```python
from build123d import *

# Parameters (mm, degrees)
BOSS_EXTRUDE1_DEPTH = 10.5
SKETCH4_W           = 30.5
SKETCH4_H           = 6
BOSS_EXTRUDE2_DEPTH = 5
SKETCH5_W           = 30.5
SKETCH5_H           = 6
BOSS_EXTRUDE3_DEPTH = 6
SKETCH6_R           = 6
CUT_EXTRUDE2_DEPTH  = 5
SKETCH11_W          = 30.5
SKETCH11_H          = 6
BOSS_EXTRUDE5_DEPTH = 15
CUT_EXTRUDE4_DEPTH  = 31.5


with BuildPart() as part:
    # Sketch2 → Boss-Extrude1 (new body)
    with BuildSketch(Plane(origin=(0, 0, 0), x_dir=(0, 0, -1), z_dir=(1, 0, 0))):
        with BuildLine():
            Line((2.711841856, 20.960264901), (-3.288158144, 20.960264901))
            Line((-3.288158144, 20.960264901), (-3.288158144, 11.676412171))
            ThreePointArc((-3.288158144, 11.676412171), (-14.220841983, 11.857208885), (-15.122437882, 0.960264901))
            Line((-15.122437882, 0.960264901), (-33.288158144, 0.960264901))
            Line((-33.288158144, 0.960264901), (-33.288158144, -5.039735099))
            Line((-33.288158144, -5.039735099), (2.711841856, -5.039735099))
            Line((2.711841856, -5.039735099), (2.711841856, 20.960264901))
        make_face()
    extrude(amount=-BOSS_EXTRUDE1_DEPTH)

    # Sketch4 → Boss-Extrude2 (add)
    with BuildSketch(Plane(origin=(0, 20.960264901, 0), x_dir=(1, 0, 0), z_dir=(0, 1, 0))):
        with Locations((4.75, -0.288158144)):
            Rectangle(SKETCH4_W, SKETCH4_H)
    extrude(amount=BOSS_EXTRUDE2_DEPTH)

    # Sketch5 → Boss-Extrude3 (add)
    with BuildSketch(Plane.XY.offset(33.288158144)):
        with Locations((4.75, -2.039735099)):
            Rectangle(SKETCH5_W, SKETCH5_H)
    extrude(amount=BOSS_EXTRUDE3_DEPTH)

    # Sketch6 → Cut-Extrude2 (cut)
    with BuildSketch(Plane(origin=(0, 0, 0), x_dir=(0, 0, -1), z_dir=(1, 0, 0))):
        with Locations((-8.806939463, 5.923867659)):
            Circle(SKETCH6_R)
    extrude(amount=-CUT_EXTRUDE2_DEPTH, mode=Mode.SUBTRACT)

    # Sketch11 → Boss-Extrude5 (add)
    with BuildSketch(Plane(origin=(0, 0.960264901, 0), x_dir=(1, 0, 0), z_dir=(0, 1, 0))):
        with Locations((4.75, -36.288158144)):
            Rectangle(SKETCH11_W, SKETCH11_H)
    extrude(amount=BOSS_EXTRUDE5_DEPTH)

    # Sketch12 → Cut-Extrude4 (cut, through all)
    with BuildSketch(Plane.ZY.offset(10.5)):
        Polygon((33.288158144, 15.960264901), (39.288158144, 15.960264901), (33.288158144, 12.496163286), align=None)
    extrude(amount=-CUT_EXTRUDE4_DEPTH, mode=Mode.SUBTRACT)


solid = part.part
```
The model under review builds one solid part; all positions refer to its coordinate system, in mm. A direction names the side the tool comes from. Coordinates: 2 decimals unless noted, no trailing zeros. Order: outer loops, then holes, each group sorted by start corner. A loop starts at its lowest first (then second) coordinate and runs counter-clockwise, first axis right, second up. Notation, with made-up numbers: (59, 42.5) -> (114, 42.5) arc R16 ccw to (114, 61.5) -> close; hole circle Ø4 at (-18.75, 47.25). An arc over 180 degrees is marked (long way). Answer in a Markdown table with one row per item. Add a question column.
Item 1: Clearance check with flat-ended pins moving along their axes: pin 1 (7 mm diameter, centred on y = 5.92, z = 8.81, fed in from +X); pin 2 (8.5 mm diameter, centred on x = -3.5, z = 20, fed in from +Y); pin 3 (1.8 mm diameter, centred on x = 8.5, z = 1.5, fed in from -Y). State where each tip first meets the part, or that it passes through.
Item 2: We need section B-B on y = 1.5. Write out the cut boundary in (x, z).
Item 3: We need section A-A on x = 6.5. Write out the cut boundary in (y, z), plus the area to 3 significant figures.
Item 4: Mouldability with a two-part tool opening along Z and no side actions: class faces 5 (the flat face through (5, 25.96, 0)), 6 (the flat face through (-2, 14, -2.712)), 7 (the flat face through (4.536, 14.252, 36.33)), 8 (the cylindrical face through (-5.176, 11.969, 14.095)) as +Z half, -Z half, draft (parallel to the pull), parting line (faces both ways), or undercut.
Item 5: To check wall thickness, follow probe 1 along Y at (x, z) = (-6, 30); probe 2 along X at (y, z) = (2, 5.5); probe 3 along Z at (x, y) = (5, 22). State the ranges of each line that lie inside material, in increasing order.
Item 6: Machinability: for faces 1 (the flat face through (10, 20.96, 0)), 2 (the flat face through (5, 4, 33.288)), 3 (the cylindrical face through (-2.46, 10.98, 5.58)), 4 (the flat face through (0, -1, 12)), which of the approach directions +Z, -Z, +X, -X, +Y, -Y give a long, thin tool a straight path to every point of the face, cutting with its end or side? Answer none if there is none.
Item 7: We need section D-D on y = 13. Write out the cut boundary in (x, z).
Item 8: We need section C-C on z = 6.5. Write out the cut boundary in (x, y), plus the area to 3 significant figures.
Final values:
| question | item | result |
|---|---|---|
| 1 | pin 1 | stops at x = -5 |
| 1 | pin 2 | stops at y = 9.98 |
| 1 | pin 3 | stops at y = 20.96 |
| 2 | outline | (-10.5, -2.71) -> (0, -2.71) -> (0, 4.75) -> (-5, 4.75) -> (-5, 12.86) -> (0, 12.86) -> (0, 15.51) -> (-10.5, 15.51) -> close; (-10.5, 33.29) -> (20, 33.29) -> (20, 39.29) -> (-10.5, 39.29) -> close |
| 3 | outline | (-5.04, 33.29) -> (12.5, 33.29) -> (15.96, 39.29) -> (-5.04, 39.29) -> close; (20.96, -2.71) -> (25.96, -2.71) -> (25.96, 3.29) -> (20.96, 3.29) -> close |
| 3 | area | 146 mm2 |
| 4 | face 5 | draft |
| 4 | face 6 | -Z half |
| 4 | face 7 | undercut |
| 4 | face 8 | undercut |
| 5 | probe 1 | y = -5.04 to 0.96 |
| 5 | probe 2 | x = -10.5 to -5 |
| 5 | probe 3 | z = -2.71 to 3.29 |
| 6 | face 1 | +Z, -Z, +X, -Y |
| 6 | face 2 | +X, +Y |
| 6 | face 3 | +X |
| 6 | face 4 | -Z, +X, -Y |
| 7 | outline | (-10.5, -2.71) -> (0, -2.71) -> (0, 3.29) -> (-10.5, 3.29) -> close; (-10.5, 5.11) -> (0, 5.11) -> (0, 12.59) -> (-10.5, 12.59) -> close; (-10.5, 34.16) -> (20, 34.16) -> (20, 39.29) -> (-10.5, 39.29) -> close |
| 8 | outline | (-10.5, -5.04) -> (0, -5.04) -> (0, 0.39) -> (-5, 0.39) -> (-5, 11.46) -> (0, 11.46) -> (0, 13.57) -> (-10.5, 13.57) -> close |
| 8 | area | 140 mm2 |
